```python
from build123d import *

# Parameters (mm, degrees)
ESQUISSE1_W                         = 7
ESQUISSE1_H                         = 4
BOSS_EXTRU_1_DEPTH                  = 200
ENL_V_MAT_EXTRU_1_DEPTH             = 5
ESQUISSE5_R                         = 1
ENL_V_MAT_EXTRU_3_DEPTH             = 1
ENL_V_MAT_EXTRU_3_DIRECTION_2_REACH = 202
CONG_6_R                            = 0.3


with BuildPart() as part:
    # Esquisse1 → Boss.-Extru.1 (new body)
    with BuildSketch(Plane.XY):
        Rectangle(ESQUISSE1_W, ESQUISSE1_H)
    extrude(amount=BOSS_EXTRU_1_DEPTH)

    # Esquisse2 → Enlèv. mat.-Extru.1 (cut, through all)
    with BuildSketch(Plane(origin=(0, 2, 0), x_dir=(1, 0, 0), z_dir=(0, 1, 0))):
        with BuildLine():
            Line((-1.65, -190), (-1.65, -10))
            ThreePointArc((-1.65, -10), (0, -8.35), (1.65, -10))
            Line((1.65, -10), (1.65, -190))
            ThreePointArc((1.65, -190), (0, -191.65), (-1.65, -190))
        make_face()
    extrude(amount=-ENL_V_MAT_EXTRU_1_DEPTH, mode=Mode.SUBTRACT)

    # Esquisse5 → Enlèv. mat.-Extru.3 (cut)
    with BuildSketch(Plane.XY.offset(200)):
        Circle(ESQUISSE5_R)
    extrude(amount=ENL_V_MAT_EXTRU_3_DEPTH, mode=Mode.SUBTRACT)

    # Esquisse5 → Enlèv. mat.-Extru.3 direction 2 (cut, up to next)
    with BuildSketch(Plane.XY.offset(200), mode=Mode.PRIVATE) as enl_v_mat_extru_3_direction_2_sk1:
        Circle(ESQUISSE5_R)
    enl_v_mat_extru_3_direction_2_tool1 = extrude(enl_v_mat_extru_3_direction_2_sk1.sketch, amount=-ENL_V_MAT_EXTRU_3_DIRECTION_2_REACH, mode=Mode.PRIVATE) & part.part
    add(enl_v_mat_extru_3_direction_2_tool1.solids().sort_by_distance((0, 0, 200))[0], mode=Mode.SUBTRACT)

    # Congé6
    cong_6_edges = [part.edges().sort_by_distance(p)[0] for p in [
        (-3.5, -2, 100),
        (0, -2, 0),
        (0, -2, 200),
        (3.5, -2, 100),
        (0, -2, 191.65),
        (1.65, -2, 100),
        (0, -2, 8.35),
        (-1.65, -2, 100),
        (-3.5, 2, 100),
        (-3.5, 0, 0),
        (-3.5, 0, 200),
        (3.5, 0, 0),
        (0, 2, 0),
        (3.5, 0, 200),
        (0, 2, 200),
        (-1, 0, 200),
        (3.5, 2, 100),
        (0, 2, 191.65),
        (1.65, 2, 100),
        (0, 2, 8.35),
        (-1.65, 2, 100),
    ]]
    fillet(cong_6_edges, radius=CONG_6_R)


solid = part.part
```
Geometry: final body of the model. Coordinates: model frame, mm. A direction names the side the tool comes from. Give positions to 0.01 mm unless a question says otherwise; leave off trailing zeros. Order: outer loops, then holes, each group sorted by start corner. A loop starts at its lowest first (then second) coordinate and runs counter-clockwise, first axis right, second up. Notation, with made-up numbers: (53.25, 2.5) -> (74.25, 2.5) arc R21 ccw to (74.25, 18.5) -> close; hole circle Ø11 at (1, -39.5). An arc over 180 degrees is marked (long way). Write each question's results on one line, items separated by ' | '. Start each with the question number.
1) First-contact query: pin 1 (1.6 mm diameter, centred on x = 0, y = 0, fed in from +Z). Flat tip, straight axial feed; report the tip coordinate or a pass-through.
2) Section B-B (y = 0). Return loops of the section in (x, z).
3) Draft query along Z for faces 1 (the flat face through (-1.65, 0, 101)), 2 (the flat face through (-2.2, -2, 98.6)), 3 (the flat face through (0, 0, 0)). Return one class per face: pulls with the +Z half, pulls with the -Z half, needs draft (parallel to the pull), parting line crosses it, or undercut.
4) Section A-A (z = 103). Return loops of the section in (x, y).
5) Set-up query: faces 4 (the flat face through (1.65, 0, 99)), 5 (the flat face through (-3.5, 0, 99)). Return all of +Z, -Z, +X, -X, +Y, -Y with unobstructed straight access to the full face (end or side cutting, diameter ignored); none if empty.
6) Line query: line 1 (Y direction, x = 0, z = 196.5); line 2 (X direction, y = 0.1, z = 137); line 3 (X direction, y = 0, z = 193.75). Output: solid intervals per line, ascending. Write a range as from..to.
Calculated:
1) pin 1: z = 8.56
2) outline: (-3.5, 0.3) arc R0.3 ccw to (-3.2, 0) -> (3.2, 0) arc R0.3 ccw to (3.5, 0.3) -> (3.5, 199.7) arc R0.3 ccw to (3.2, 200) -> (1.3, 200) arc R0.3 ccw to (1, 199.7) -> (1, 191.31) arc R1.65 cw to (1.65, 190) -> (1.65, 10) arc R1.65 cw to (-1.65, 10) -> (-1.65, 190) arc R1.65 cw to (-1, 191.31) -> (-1, 199.7) arc R0.3 ccw to (-1.3, 200) -> (-3.2, 200) arc R0.3 ccw to (-3.5, 199.7) -> close
3) face 1: undercut | face 2: needs draft | face 3: pulls with the -Z half
4) outline: (-3.5, -1.7) arc R0.3 ccw to (-3.2, -2) -> (-1.95, -2) arc R0.3 ccw to (-1.65, -1.7) -> (-1.65, 1.7) arc R0.3 ccw to (-1.95, 2) -> (-3.2, 2) arc R0.3 ccw to (-3.5, 1.7) -> close; (1.65, -1.7) arc R0.3 ccw to (1.95, -2) -> (3.2, -2) arc R0.3 ccw to (3.5, -1.7) -> (3.5, 1.7) arc R0.3 ccw to (3.2, 2) -> (1.95, 2) arc R0.3 ccw to (1.65, 1.7) -> close
5) face 4: +Y, -Y | face 5: +Z, -Z, -X, +Y, -Y
6) line 1: -2..-1, 1..2 | line 2: -3.5..-1.65, 1.65..3.5 | line 3: -3.5..-1, 1..3.5
